```python
from build123d import *

# Parameters (mm, degrees)
F0_W      = 88.9
F0_H      = 40.64
F1_DEPTH  = 35.56
F3_DEPTH  = 7.62
F5_DEPTH  = 7.62
F7_DEPTH  = 36.322
F9_DEPTH  = 9.906
F11_DEPTH = 6.35
F13_DEPTH = 9.144
F14_R     = 3.81
F15_DEPTH = 6.604
F16_R     = 3.297802
F16_R_2   = 3.302
F17_DEPTH = 4.572
F18_R     = 3.679261


with BuildPart() as f1:
    # F0 (on Front) → F1 (new body)
    with BuildSketch(Plane.XZ):
        with Locations((1.685638, 1.512455)):
            Rectangle(F0_W, F0_H)
    extrude(amount=F1_DEPTH)

    # F2 (on face) → F3 (join)
    with BuildSketch(Plane.XZ.offset(35.56)):
        with BuildLine():
            Line((-20.58096, -18.807545), (-38.36096, -18.807545))
            ThreePointArc((-38.36096, -18.807545), (-29.47096, -27.697545), (-20.58096, -18.807545))
        make_face()
        with BuildLine():
            Line((40.796571, -18.807545), (23.016571, -18.807545))
            ThreePointArc((23.016571, -18.807545), (31.906571, -27.697545), (40.796571, -18.807545))
        make_face()
    extrude(amount=-F3_DEPTH)

    # F4 (on face) → F5 (join)
    with BuildSketch(Plane(origin=(0, 0, 0), x_dir=(-1, 0, 0), z_dir=(0, 1, 0))):
        with BuildLine():
            Line((-23.503698, -18.807545), (-41.283698, -18.807545))
            ThreePointArc((-41.283698, -18.807545), (-32.393698, -27.697545), (-23.503698, -18.807545))
        make_face()
        with BuildLine():
            Line((38.604519, -18.807545), (20.824519, -18.807545))
            ThreePointArc((20.824519, -18.807545), (29.714519, -27.697545), (38.604519, -18.807545))
        make_face()
    extrude(amount=-F5_DEPTH)

    # F6 (on face) → F7 (join)
    with BuildSketch(Plane.XZ.offset(35.56)):
        with BuildLine():
            Line((-24.699327, 21.832455), (43.047176, 21.832455))
            ThreePointArc((43.047176, 21.832455), (9.173924, 55.705706), (-24.699327, 21.832455))
        make_face()
    extrude(amount=-F7_DEPTH)

    # F8 (on face) → F9 (join)
    with BuildSketch(Plane.XZ.offset(35.56)):
        with BuildLine():
            Line((-18.899895, 24.207648), (34.604043, 24.207648))
            ThreePointArc((34.604043, 24.207648), (7.852074, 50.959617), (-18.899895, 24.207648))
        make_face()
    extrude(amount=-F9_DEPTH)

    # F10 (on face) → F11 (cut)
    with BuildSketch(Plane.XZ.offset(35.56)):
        with BuildLine():
            Line((-19.053006, 21.832455), (37.400854, 21.832455))
            ThreePointArc((37.400854, 21.832455), (9.173924, 50.059384), (-19.053006, 21.832455))
        make_face()
    extrude(amount=-F11_DEPTH, mode=Mode.SUBTRACT)

    # F12 (on face) → F13 (cut)
    with BuildSketch(Plane(origin=(0, 0.762, 0), x_dir=(-1, 0, 0), z_dir=(0, 1, 0))):
        with BuildLine():
            Line((-39.26131, 21.832455), (20.913462, 21.832455))
            ThreePointArc((20.913462, 21.832455), (-9.173924, 51.919841), (-39.26131, 21.832455))
        make_face()
    extrude(amount=-F13_DEPTH, mode=Mode.SUBTRACT)

    # F14 (on face) → F15 (cut)
    with BuildSketch(Plane.YZ.offset(46.135638)):
        with Locations((-27.224183, 0)):
            Circle(F14_R)
        with Locations((-9.559637, 0)):
            Circle(F14_R)
    extrude(amount=-F15_DEPTH, mode=Mode.SUBTRACT)

    # F16 (on face) → F17 (cut)
    with BuildSketch(Plane(origin=(-42.764362, 0, 0), x_dir=(0, -1, 0), z_dir=(-1, 0, 0))):
        with Locations((9.101178, 0)):
            Circle(F16_R)
        with Locations((26.068604, 0)):
            Circle(F16_R_2)
    extrude(amount=-F17_DEPTH, mode=Mode.SUBTRACT)

    # F18
    f18_edges = [f1.edges().sort_by_distance(p)[0] for p in [
        (-29.47096, -35.56, -27.697545),
        (-29.714519, -7.62, -27.697545),
        (-29.714519, 0, -27.697545),
        (32.393698, 0, -27.697545),
        (31.906571, -27.94, -27.697545),
        (32.393698, -7.62, -27.697545),
        (-29.47096, -27.94, -27.697545),
        (31.906571, -35.56, -27.697545),
    ]]
    fillet(f18_edges, radius=F18_R)


solid = f1.part
```
The listing builds one solid part. Answer for the finished solid, in the listing's coordinates (mm). A direction names the side the tool comes from. Give positions to 0.01 mm unless a question says otherwise; leave off trailing zeros. Loops run counter-clockwise (first coordinate to the right, second up) from the corner with the lowest first, then second, coordinate; pieces in that order, holes last. Notation, with made-up numbers: (33, 44.25) - (77, 44.25) arc R26 ccw to (77, 68.25) - close; hole circle Ø8 at (88, 37). An arc over 180 degrees is marked (long way). Answer as CSV lines item,"result". Start each with the question number.
Item 1: Each of these flat-tipped pins is pushed along its axis until it touches: pin 1 (0.9 mm diameter, centred on x = 44.5, y = -24.5, fed in from +Z); pin 2 (6 mm diameter, centred on x = 4.5, y = -7, fed in from -Z); pin 3 (7 mm diameter, centred on y = -9.56, z = 0, fed in from -X); pin 4 (5 mm diameter, centred on x = 11, y = -11, fed in from +Z). Where does it stop, or does it pass through?
Item 2: A cutting plane is placed at C-C on y = -19.5. Determine the outline of the cut face in (x, z), then the cut area to 3 significant figures.
Item 3: The mould has two halves that part along Y. Classify faces 1 (the face through (10, -8.382, 34)), 2 (the face through (46.136, -18, 1)), 3 (the face through (-40.51, -5.807, 0.145)): +Y half, -Y half, draft (parallel to the pull), parting line (faces both ways), or undercut.
Item 4: A cutting plane is placed at A-A on z = 0. Determine the outline of the cut face in (x, y), then the cut area to 3 significant figures.
Item 5: For faces 4 (the face through (-30, -27.94, -21)), 5 (the face through (-38.192, -9, 0)), 6 (the face through (45, -18, 21.832)), determine the directions among +Z, -Z, +X, -X, +Y, -Y from which every point of the face is accessible in a straight line to the end or side of a thin tool.
Item 6: A cutting plane is placed at D-D on x = 5.5. Determine the outline of the cut face in (y, z).
Item 7: Find the intervals of material crossed by line 1 (Y direction, x = -35, z = -19); line 2 (Y direction, x = -30.5, z = -17); line 3 (X direction, y = -30.5, z = 35), in increasing order. Write a range as from..to.
Found:
1,pin 1,"stops at z = 21.83"
1,pin 2,"stops at z = -18.81"
1,pin 3,"stops at x = -42.76"
1,pin 4,"stops at z = 55.71"
2,outline,"(-42.76, -18.81) - (46.14, -18.81) - (46.14, 21.83) - (43.05, 21.83) arc R33.87 ccw to (-24.7, 21.83) - (-42.76, 21.83) - close"
2,area,"5,420 mm^2"
3,face 1,"+Y half"
3,face 2,"draft"
3,face 3,"undercut"
4,outline,"(-42.76, -35.56) - (46.14, -35.56) - (46.14, -31.03) - (39.53, -31.03) - (39.53, -23.41) - (46.14, -23.41) - (46.14, -13.37) - (39.53, -13.37) - (39.53, -5.75) - (46.14, -5.75) - (46.14, 0) - (-42.76, 0) - (-42.76, -5.8) - (-38.19, -5.8) - (-38.19, -12.4) - (-42.76, -12.4) - (-42.76, -22.77) - (-38.19, -22.77) - (-38.19, -29.37) - (-42.76, -29.37) - close"
4,area,"3,000 mm^2"
5,face 4,"-Z, +X, -X"
5,face 5,"-X"
5,face 6,"+Z, +X, +Y, -Y"
6,outline,"(-35.56, -18.81) - (0, -18.81) - (0, 21.83) - (-8.38, 21.83) - (-8.38, 51.69) - (0.76, 51.69) - (0.76, 55.51) - (-35.56, 55.51) - (-35.56, 49.82) - (-29.21, 49.82) - (-29.21, 21.83) - (-35.56, 21.83) - close"
7,line 1,"y = -35.55..-27.95, -7.62..0"
7,line 2,"y = -35.56..0"
7,line 3,"x = -22.04..-15.79, 34.14..40.38"
